Geometry: final body of the model. Coordinates: model frame, mm. A direction names the side the tool comes from. Give positions to 0.01 mm unless a question says otherwise; leave off trailing zeros. Write each loop counter-clockwise with the first axis right and the second up, starting at its lowest first coordinate (ties: lowest second). Pieces come first, ordered by that corner, then holes. Notation, with made-up numbers: M 81.5,58.25 L 125.5,58.25 A20 ccw 125.5,92.25 Z; hole C -11,-2.5 d8. An arc over 180 degrees is marked long. Use a Markdown table: item, result. Add a question column.
1) Section A-A on x = 0. Return the cut outline in (y, z), then the cut area to 3 significant figures.
2) Line query: line 1 (Y direction, x = 0, z = 12); line 2 (Z direction, x = 25, y = 0); line 3 (Z direction, x = 0, y = -23). Output: solid intervals per line, ascending.
3) Section C-C on z = 18.5. Return the cut outline in (x, y), then the cut area to 3 significant figures.
4) Draft query along Y for faces 1 (the flat face through (-6.5, -23.3, 0)), 2 (the flat face through (-10.3, -10.3, 25)), 3 (the cylindrical face through (13.38, -25.73, 23.67)). Return one class per face: +Y half, -Y half, draft (parallel to the pull), parting line (faces both ways), or undercut.
5) Set-up query: faces 4 (the cylindrical face through (23.977, 1.055, 12.325)), 5 (the cylindrical face through (-13.986, 0.616, 36.657)), 6 (the cylindrical face through (21, 0, 44)). Return all of +Z, -Z, +X, -X, +Y, -Y with unobstructed straight access to the full face (end or side cutting, diameter ignored); none if empty.
6) Section B-B on y = 0. Return the cut outline in (x, z).
7) Pin query (flat end, axial travel): pin 1 (3 mm diameter, centred on y = -8.5, z = 10.5, fed in from -X); pin 2 (3 mm diameter, centred on y = 19.5, z = 29.5, fed in from +X); pin 3 (25 mm diameter, centred on x = 0, y = 0, fed in from -Z); pin 4 (10 mm diameter, centred on x = -22, y = -21, fed in from +Z). Return the tip coordinate at first contact, or that it passes through.
8) Section D-D on z = 39. Return the cut outline in (x, y).
```python
from build123d import *

# Parameters (mm, degrees)
SKETCH4_R               = 29
BOSS_EXTRUDE1_DEPTH     = 48
SKETCH5_R               = 24
CUT_EXTRUDE1_DEPTH      = 25
SKETCH6_R               = 14
CUT_EXTRUDE2_DEPTH      = 1
CUT_EXTRUDE2_DEPTH_BACK = 49
SKETCH7_R               = 5
CUT_EXTRUDE3_DEPTH      = 42
FILLET1_R               = 0.3


with BuildPart() as part:
    # Sketch4 → Boss-Extrude1 (new body)
    with BuildSketch(Plane.XY):
        Circle(SKETCH4_R)
    extrude(amount=BOSS_EXTRUDE1_DEPTH)

    # Sketch5 → Cut-Extrude1 (cut)
    with BuildSketch(Plane(origin=(0, 0, 0), x_dir=(-1, 0, 0), z_dir=(0, 0, -1))):
        Circle(SKETCH5_R)
    extrude(amount=-CUT_EXTRUDE1_DEPTH, mode=Mode.SUBTRACT)

    # Sketch6 → Cut-Extrude2 (cut, two sides)
    with BuildSketch(Plane.XY.offset(48)) as cut_extrude2_sk:
        Circle(SKETCH6_R)
    extrude(amount=CUT_EXTRUDE2_DEPTH, mode=Mode.SUBTRACT)
    extrude(cut_extrude2_sk.sketch, amount=-CUT_EXTRUDE2_DEPTH_BACK, mode=Mode.SUBTRACT)

    # Sketch7 → Cut-Extrude3 (cut)
    with BuildSketch(Plane(origin=(0, 0, 0), x_dir=(0, 0, -1), z_dir=(1, 0, 0))):
        with Locations((-39, 0)):
            Circle(SKETCH7_R)
    extrude(amount=CUT_EXTRUDE3_DEPTH, mode=Mode.SUBTRACT)

    # Fillet1
    fillet1_edges = [part.edges().sort_by_distance(p)[0] for p in [
        (-14, 0, 48),
        (-14, 0, 25),
        (-29, 0, 0),
        (-29, 0, 48),
    ]]
    fillet(fillet1_edges, radius=FILLET1_R)


solid = part.part
```
Found:
| question | item | result |
|---|---|---|
| 1 | outline | M -29,0.3 A0.3 ccw -28.7,0 L -24,0 L -24,25 L -14.3,25 A0.3 ccw -14,25.3 L -14,47.7 A0.3 ccw -14.3,48 L -28.7,48 A0.3 ccw -29,47.7 Z; M 14,25.3 A0.3 ccw 14.3,25 L 24,25 L 24,0 L 28.7,0 A0.3 ccw 29,0.3 L 29,47.7 A0.3 ccw 28.7,48 L 14.3,48 A0.3 ccw 14,47.7 Z |
| 1 | area | 940 mm² |
| 2 | line 1 | -29 to -24, 24 to 29 |
| 2 | line 2 | 0 to 34, 44 to 48 |
| 2 | line 3 | 25 to 48 |
| 3 | outline | C 0,0 d58; hole C 0,0 d48 |
| 3 | area | 833 mm² |
| 4 | face 1 | draft |
| 4 | face 2 | undercut |
| 4 | face 3 | parting line |
| 5 | face 4 | -Z |
| 5 | face 5 | +Z, -Z |
| 5 | face 6 | +X |
| 6 | outline | M -29,0.3 A0.3 ccw -28.7,0 L -24,0 L -24,25 L -14.3,25 A0.3 ccw -14,25.3 L -14,47.7 A0.3 ccw -14.3,48 L -28.7,48 A0.3 ccw -29,47.7 Z; M 14,25.3 A0.3 ccw 14.3,25 L 24,25 L 24,0 L 28.7,0 A0.3 ccw 29,0.3 L 29,34 L 14,34 Z; M 14,44 L 29,44 L 29,47.7 A0.3 ccw 28.7,48 L 14.3,48 A0.3 ccw 14,47.7 Z |
| 7 | pin 1 | x = -28.14 |
| 7 | pin 2 | x = 22.74 |
| 7 | pin 3 | through |
| 7 | pin 4 | z = 48 |
| 8 | outline | M 13.08,-5 A14 cw long 13.08,5 L 28.57,5 A29 ccw long 28.57,-5 Z |
